from build123d import *

# Parameters (mm, degrees)
SKETCH_1_R          = 3.25
SKETCH_1_R_2        = 7.5
EXTRUDE_1_DEPTH     = 6
SKETCH_2_W          = 1
SKETCH_2_H          = 19.943647813
CUT_EXTRUDE_1_DEPTH = 36.578503871
CHAMFER_1_SIZE      = 5.5
CHAMFER_2_SIZE      = 0.5


with BuildPart() as part:
    # Эскиз1 → Бобышка-Вытянуть1 (new body)
    with BuildSketch(Plane.XY):
        with BuildLine():
            Line((15, 60.126164395), (15, 400))
            Line((15, 400), (-15, 400))
            Line((-15, 400), (-15, 60.126164395))
            ThreePointArc((-15, 60.126164395), (-11.99467632, 46.284317121), (-16.512069377, 32.859643332))
            ThreePointArc((-16.512069377, 32.859643332), (0, 0), (16.512069377, 32.859643332))
            ThreePointArc((16.512069377, 32.859643332), (11.99467632, 46.284317121), (15, 60.126164395))
        make_face()
        with Locations((0, 370)):
            Circle(SKETCH_1_R, mode=Mode.SUBTRACT)
        with Locations((0, 350)):
            Circle(SKETCH_1_R, mode=Mode.SUBTRACT)
        with Locations((0, 20.578503871)):
            Circle(SKETCH_1_R_2, mode=Mode.SUBTRACT)
    extrude(amount=EXTRUDE_1_DEPTH)

    # Эскиз2 → Вырез-Вытянуть1 (cut, through all)
    with BuildSketch(Plane.ZY.offset(15)):
        with Locations((5.5, 390.028176094)):
            Rectangle(SKETCH_2_W, SKETCH_2_H)
    extrude(amount=-CUT_EXTRUDE_1_DEPTH, mode=Mode.SUBTRACT)

    # Фаска1
    chamfer_1_edges = [part.edges().sort_by_distance(p)[0] for p in [
        (-3.25, 370, 0),
    ]]
    chamfer(chamfer_1_edges, length=CHAMFER_1_SIZE)

    # Фаска2
    chamfer_2_edges = [part.edges().sort_by_distance(p)[0] for p in [
        (-3.25, 350, 0),
        (-3.25, 350, 6),
    ]]
    chamfer(chamfer_2_edges, length=CHAMFER_2_SIZE)


solid = part.part
Could you check a few things on this model? Use its own coordinates, in mm. A direction names the side the tool comes from. Coordinates: 2 decimals unless noted, no trailing zeros. Write each loop counter-clockwise with the first axis right and the second up, starting at its lowest first coordinate (ties: lowest second). Pieces come first, ordered by that corner, then holes. Notation, with made-up numbers: (48, 1.5) - (90, 1.5) arc R16 ccw to (90, 20.5) - close; hole circle Ø9 at (22.25, -32.5). An arc over 180 degrees is marked (long way). Put each result on its own line as item: value. Start each with the question number.
Q1. I want a section at C-C on y = 293. Write out the boundary of the cut face in (x, z).
Q2. I want a section at B-B on y = 370. Write out the boundary of the cut face in (x, z), plus the area to 3 significant figures.
Q3. Which directions (+Z, -Z, +X, -X, +Y, -Y) give clear straight access to the entire face, cutting with the end or side of a thin tool? Please do faces 4 (the cylindrical face through (-1.626, 13.257, 2.958)), 5 (the flat face through (0, 390, 5)).
Q4. Thinking about a two-plate mould opening in Y: for faces 1 (the cylindrical face through (-0.64, 0.01, 2.96)), 2 (the flat face through (0, 203, 0)), 3 (the cylindrical face through (-0.705, 346.827, 2.965)), which applies, pulls with the +Y half, pulls with the -Y half, needs draft (parallel to the pull), parting line crosses it, or undercut?
Q5. I want a section at A-A on x = 0. Write out the boundary of the cut face in (y, z), plus the area to 3 significant figures.
Q6. Please list where these lines run through material, in increasing order: L1, parallel to Y at x = 0, z = 5.95; L2, parallel to X at y = 370, z = 5.85; L3, parallel to Y at x = 0, z = 5.7.
Q7. I'm going to push flat-ended pins straight in: P1, Ø1, axis at y = 206.5, z = 3.5, coming from the +X side; P2, Ø1, axis at x = 12, z = 3.5, coming from the -Y side; P3, Ø24, axis at x = 0, y = 20.58, coming from the +Z side; P4, Ø1.8, axis at y = 282.5, z = 4.5, coming from the -X side. Where does each tip first touch, or does it pass through?
Checks:
1. outline: (-15, 0) - (15, 0) - (15, 6) - (-15, 6) - close
2. outline: (-15, 0) - (-8.75, 0) - (-3.25, 5.5) - (-3.25, 6) - (-15, 6) - close; (3.25, 5.5) - (8.75, 0) - (15, 0) - (15, 6) - (3.25, 6) - close
2. area: 111 mm²
3. face 4: +Z, -Z
3. face 5: +Z, +X, -X, +Y
4. face 1: parting line crosses it
4. face 2: needs draft
4. face 3: undercut
5. outline: (0, 0) - (13.08, 0) - (13.08, 6) - (0, 6) - close; (28.08, 0) - (346.25, 0) - (346.75, 0.5) - (346.75, 5.5) - (346.25, 6) - (28.08, 6) - close; (353.25, 0.5) - (353.75, 0) - (361.25, 0) - (366.75, 5.5) - (366.75, 6) - (353.75, 6) - (353.25, 5.5) - close; (373.25, 5.5) - (378.75, 0) - (400, 0) - (400, 5) - (380.06, 5) - (380.06, 6) - (373.25, 6) - close
5. area: 2,180 mm²
6. L1: 0 to 13.08, 28.08 to 346.3, 353.7 to 366.75, 373.25 to 380.06
6. L2: -15 to -3.25, 3.25 to 15
6. L3: 0 to 13.08, 28.08 to 346.55, 353.45 to 366.75, 373.25 to 380.06
7. P1: x = 15
7. P2: y = 3.51
7. P3: z = 6
7. P4: x = -15
